```python
from build123d import *

# Parameters (mm, degrees)
BOSS_EXTRUDE1_DEPTH = 10
SKETCH4_R           = 3
BOSS_EXTRUDE2_DEPTH = 4
CUT_EXTRUDE2_DEPTH  = 10
SKETCH9_R           = 5
CUT_EXTRUDE3_DEPTH  = 15
SKETCH10_R          = 6.98
SKETCH10_R_2        = 5
BOSS_EXTRUDE3_DEPTH = 7
SKETCH11_R          = 1.5
CUT_EXTRUDE4_DEPTH  = 21


with BuildPart() as part:
    # Sketch3 → Boss-Extrude1 (new body)
    with BuildSketch(Plane.XY):
        with BuildLine():
            Line((-7.72865, 2.586593), (-6.793519, 2.323899))
            ThreePointArc((-6.793519, 2.323899), (-7.18, 0), (-6.793519, -2.323899))
            Line((-6.793519, -2.323899), (-7.72865, -2.586593))
            ThreePointArc((-7.72865, -2.586593), (-7.058107, -4.075), (-6.104381, -5.399911))
            Line((-6.104381, -5.399911), (-5.409315, -4.72141))
            ThreePointArc((-5.409315, -4.72141), (-3.59, -6.218062), (-1.384204, -7.045309))
            Line((-1.384204, -7.045309), (-1.62427, -7.986504))
            ThreePointArc((-1.62427, -7.986504), (0, -8.15), (1.62427, -7.986504))
            Line((1.62427, -7.986504), (1.384204, -7.045309))
            ThreePointArc((1.384204, -7.045309), (3.59, -6.218062), (5.409315, -4.72141))
            Line((5.409315, -4.72141), (6.104381, -5.399911))
            ThreePointArc((6.104381, -5.399911), (7.058107, -4.075), (7.72865, -2.586593))
            Line((7.72865, -2.586593), (6.793519, -2.323899))
            ThreePointArc((6.793519, -2.323899), (7.18, 0), (6.793519, 2.323899))
            Line((6.793519, 2.323899), (7.72865, 2.586593))
            ThreePointArc((7.72865, 2.586593), (7.058107, 4.075), (6.104381, 5.399911))
            Line((6.104381, 5.399911), (5.409315, 4.72141))
            ThreePointArc((5.409315, 4.72141), (3.59, 6.218062), (1.384204, 7.045309))
            Line((1.384204, 7.045309), (1.62427, 7.986504))
            ThreePointArc((1.62427, 7.986504), (0, 8.15), (-1.62427, 7.986504))
            Line((-1.62427, 7.986504), (-1.384204, 7.045309))
            ThreePointArc((-1.384204, 7.045309), (-3.59, 6.218062), (-5.409315, 4.72141))
            Line((-5.409315, 4.72141), (-6.104381, 5.399911))
            ThreePointArc((-6.104381, 5.399911), (-7.058107, 4.075), (-7.72865, 2.586593))
        make_face()
    extrude(amount=BOSS_EXTRUDE1_DEPTH)

    # Sketch4 → Boss-Extrude2 (add)
    with BuildSketch(Plane(origin=(0, 0, 0), x_dir=(-1, 0, 0), z_dir=(0, 0, -1))):
        with BuildLine():
            Line((-15, 10), (15, 10))
            ThreePointArc((15, 10), (25, 0), (15, -10))
            Line((15, -10), (-15, -10))
            ThreePointArc((-15, -10), (-25, 0), (-15, 10))
        make_face()
        with Locations((-15, 0)):
            Circle(SKETCH4_R, mode=Mode.SUBTRACT)
        with Locations((15, 0)):
            Circle(SKETCH4_R, mode=Mode.SUBTRACT)
    extrude(amount=BOSS_EXTRUDE2_DEPTH)

    # Sketch8 → Cut-Extrude2 (cut)
    with BuildSketch(Plane.XY.offset(10)):
        with BuildLine():
            Line((-5.409315, 4.72141), (-5.258637, 4.589895))
            ThreePointArc((-5.258637, 4.589895), (-3.49, 6.044857), (-1.345647, 6.849061))
            Line((-1.345647, 6.849061), (-1.384204, 7.045309))
            ThreePointArc((-1.384204, 7.045309), (-3.59, 6.218062), (-5.409315, 4.72141))
        make_face()
        with BuildLine():
            Line((5.409315, 4.72141), (5.258637, 4.589895))
            ThreePointArc((5.258637, 4.589895), (3.49, 6.044857), (1.345647, 6.849061))
            Line((1.345647, 6.849061), (1.384204, 7.045309))
            ThreePointArc((1.384204, 7.045309), (3.59, 6.218062), (5.409315, 4.72141))
        make_face()
        with BuildLine():
            Line((6.793519, -2.323899), (6.604284, -2.259166))
            ThreePointArc((6.604284, -2.259166), (6.98, 0), (6.604284, 2.259166))
            Line((6.604284, 2.259166), (6.793519, 2.323899))
            ThreePointArc((6.793519, 2.323899), (7.18, 0), (6.793519, -2.323899))
        make_face()
        with BuildLine():
            Line((1.384204, -7.045309), (1.345647, -6.849061))
            ThreePointArc((1.345647, -6.849061), (3.49, -6.044857), (5.258637, -4.589895))
            Line((5.258637, -4.589895), (5.409315, -4.72141))
            ThreePointArc((5.409315, -4.72141), (3.59, -6.218062), (1.384204, -7.045309))
        make_face()
        with BuildLine():
            Line((-5.409315, -4.72141), (-5.258637, -4.589895))
            ThreePointArc((-5.258637, -4.589895), (-3.49, -6.044857), (-1.345647, -6.849061))
            Line((-1.345647, -6.849061), (-1.384204, -7.045309))
            ThreePointArc((-1.384204, -7.045309), (-3.59, -6.218062), (-5.409315, -4.72141))
        make_face()
        with BuildLine():
            Line((-6.793519, 2.323899), (-6.604284, 2.259166))
            ThreePointArc((-6.604284, 2.259166), (-6.98, 0), (-6.604284, -2.259166))
            Line((-6.604284, -2.259166), (-6.793519, -2.323899))
            ThreePointArc((-6.793519, -2.323899), (-7.18, 0), (-6.793519, 2.323899))
        make_face()
    extrude(amount=-CUT_EXTRUDE2_DEPTH, mode=Mode.SUBTRACT)

    # Sketch9 → Cut-Extrude3 (cut, through all)
    with BuildSketch(Plane.XY.offset(10)):
        Circle(SKETCH9_R)
    extrude(amount=-CUT_EXTRUDE3_DEPTH, mode=Mode.SUBTRACT)

    # Sketch10 → Boss-Extrude3 (add)
    with BuildSketch(Plane.XY.offset(10)):
        Circle(SKETCH10_R)
        Circle(SKETCH10_R_2, mode=Mode.SUBTRACT)
    extrude(amount=BOSS_EXTRUDE3_DEPTH)

    # Sketch11 → Cut-Extrude4 (cut, through all)
    with BuildSketch(Plane(origin=(0, 10, 0), x_dir=(1, 0, 0), z_dir=(0, 1, 0))):
        with Locations((0, -13.5)):
            Circle(SKETCH11_R)
    extrude(amount=-CUT_EXTRUDE4_DEPTH, mode=Mode.SUBTRACT)


solid = part.part
```
Geometry: final body of the model. Coordinates: model frame, mm. A direction names the side the tool comes from. Round coordinates to 2 decimals unless told otherwise and drop trailing zeros. Loops run counter-clockwise (first coordinate to the right, second up) from the corner with the lowest first, then second, coordinate; pieces in that order, holes last.
Item 1: Reachability of faces 5 (the cylindrical face through (-7.07, -4.055, 4.93)), 6 (the cylindrical face through (7.07, 4.055, 4.93)), 7 (the cylindrical face through (-0.02, -8.15, 4.93)), 8 (the cylindrical face through (7.05, -4.09, 4.93)), 9 (the flat face through (-1.5, 7.5, 4.9)) from +Z, -Z, +X, -X, +Y, -Y: full face, straight path, thin tool, end or side. Return the list, or none.
Checked values:
face 5: +Z, -X, -Y
face 6: +Z, +X, +Y
face 7: +Z, -Y
face 8: +Z, +X, -Y
face 9: +Z, -X
Item 2: Section C-C, the plane x = 17. Output: boundary loops of the cut face in (y, z).
Checked values:
outline: (-9.8, -4) - (-2.24, -4) - (-2.24, 0) - (-9.8, 0) - close; (2.24, -4) - (9.8, -4) - (9.8, 0) - (2.24, 0) - close
Item 3: Section A-A, the plane z = -1. Output: boundary loops of the cut face in (x, y), plus the area to 3 significant figures.
Checked values:
outline: (-15, -10) - (15, -10) arc R10 ccw to (15, 10) - (-15, 10) arc R10 ccw to start; hole circle Ø6 at (-15, 0); hole circle Ø10 at (0, 0); hole circle Ø6 at (15, 0)
area: 779 mm2
Item 4: Mould query, pull axis Y, two halves, no side actions, for faces 1 (the flat face through (0, 8, 10)), 2 (the flat face through (1.5, 7.5, 4.9)), 3 (the flat face through (0, 10, -2)), 4 (the flat face through (1.5, -7.5, 4.9)). Classes: released by +Y, released by -Y, zero draft, split by the parting line, or undercut.
Checked values:
face 1: zero draft
face 2: undercut
face 3: released by +Y
face 4: undercut
Item 5: Section B-B, the plane y = 0. Output: boundary loops of the cut face in (x, z).
Checked values:
outline: (-25, -4) - (-18, -4) - (-18, 0) - (-25, 0) - close; (-12, -4) - (-5, -4) - (-5, 17) - (-6.98, 17) - (-6.98, 0) - (-12, 0) - close; (5, -4) - (12, -4) - (12, 0) - (6.98, 0) - (6.98, 17) - (5, 17) - close; (18, -4) - (25, -4) - (25, 0) - (18, 0) - close
Item 6: Section D-D, the plane z = 13.5. Output: boundary loops of the cut face in (x, y).
Checked values:
outline: (-1.5, -6.82) - (-1.5, -4.77) arc R5 cw to (-1.5, 4.77) - (-1.5, 6.82) arc R6.98 ccw to start; (1.5, -6.82) arc R6.98 ccw to (1.5, 6.82) - (1.5, 4.77) arc R5 cw to (1.5, -4.77) - close
Item 7: Contact query for flat-ended pins moving along their axis: P1, Ø1, axis at y = -1.5, z = 12.5, coming from the -X side; P2, Ø0.7, axis at x = -7, y = -3.5, coming from the +Z side; P3, Ø2.5, axis at x = 0, z = 13.5, coming from the +Y side; P4, Ø3, axis at x = -7.5, z = 7.5, coming from the -Y side. Output: stop coordinate, or through.
Checked values:
P1: stops at x = -6.91
P2: stops at z = 10
P3: passes through
P4: stops at y = -5.4
Item 8: Line query: L1, parallel to Z at x = 0, y = 6.4; L2, parallel to Y at x = 15, z = -1.4; L3, parallel to Z at x = 18.5, y = -7. Output: solid intervals per line, ascending.
Checked values:
L1: z = -4 to 12, 15 to 17
L2: y = -10 to -3, 3 to 10
L3: z = -4 to 0
